Here's the drawing with two shaded views (mm, measured from the low corner). I have some questions. A direction names the side the tool comes from. Coordinates: 2 decimals unless noted, no trailing zeros. Loops run counter-clockwise (first coordinate to the right, second up) from the corner with the lowest first, then second, coordinate; pieces in that order, holes last. Notation, with made-up numbers: M 68.25,22.5 L 80.25,22.5 A18 cw 80.25,43.5 Z; hole C 10.25,-10 d8. An arc over 180 degrees is marked long. Return JSON: item names as keys, results as strings. Group by question number.
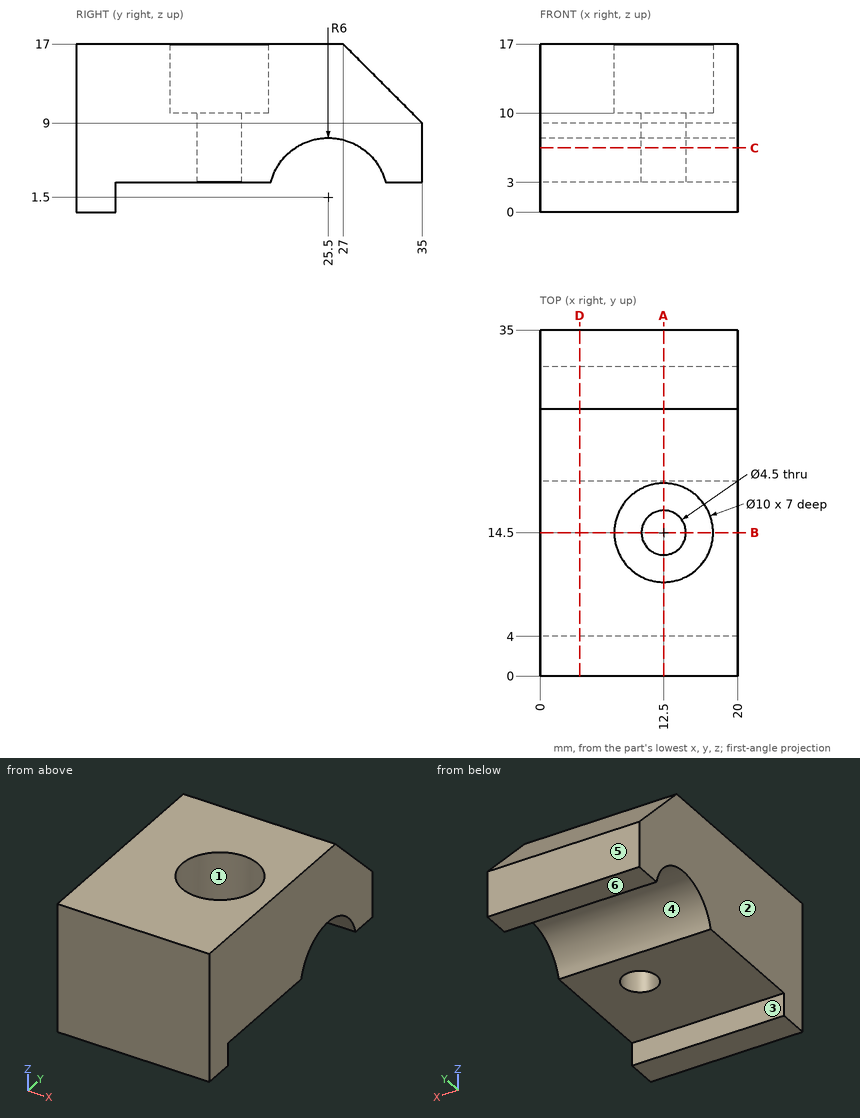
(1) Will these pins go through, and if not, where does the flat tip stop? P1, Ø3, axis at x = 15, y = 16.5, coming from the +Z side; P2, Ø4, axis at x = 9.5, y = 9, coming from the -Z side; P3, Ø3.5, axis at x = 7.5, z = 1, coming from the +Y side.
(2) If I drill on L1, parallel to Y at x = 11.25, z = 4.5; L2, parallel to Y at x = 15.5, z = 1; L3, parallel to Y at x = 18.75, z = 6.75, over which ranges is the centre line in solid material (lowest first)? Write a range as [from, to].
(3) Imagine slicing it at C-C, the plane z = 6.5. Write out the boundary of the cut face in (x, y).
(4) Imagine slicing it at D-D, the plane x = 4. Write out the boundary of the cut face in (y, z).
(5) Imagine slicing it at A-A, the plane x = 12.5. Write out the boundary of the cut face in (y, z), then the cut area to 3 significant figures.
(6) Imagine slicing it at B-B, the plane y = 14.5. Write out the boundary of the cut face in (x, z), then the cut area to 4 significant figures.
(7) We'd pull the mould along Y, two halves only. Please class the marked faces 4, 5 and 6: +Y half, -Y half, draft (parallel to the pull), parting line (faces both ways), or undercut.
(8) For the marked faces 1, 2 and 3, which set-ups out of +Z, -Z, +X, -X, +Y, -Y let a thin tool reach every point of the face, with its end or its side?
Checks:
{
 "1": {"P1": "z = 10", "P2": "z = 3", "P3": "y = 4"},
 "2": {"L1": "[0, 12.63], [16.37, 20.3], [30.7, 35]", "L2": "[0, 4]", "L3": "[0, 22.6], [28.4, 35]"},
 "3": {"outline": "M 0,0 L 20,0 L 20,22.18 L 0,22.18 Z; M 0,28.82 L 20,28.82 L 20,35 L 0,35 Z; hole C 12.5,14.5 d4.5"},
 "4": {"outline": "M 0,0 L 4,0 L 4,3 L 19.69,3 A6 cw 31.31,3 L 35,3 L 35,9 L 27,17 L 0,17 Z"},
 "5": {"outline": "M 0,0 L 4,0 L 4,3 L 12.25,3 L 12.25,10 L 9.5,10 L 9.5,17 L 0,17 Z; M 16.75,3 L 19.69,3 A6 cw 31.31,3 L 35,3 L 35,9 L 27,17 L 19.5,17 L 19.5,10 L 16.75,10 Z", "area": "330 mm²"},
 "6": {"outline": "M 0,3 L 10.25,3 L 10.25,10 L 7.5,10 L 7.5,17 L 0,17 Z; M 14.75,3 L 20,3 L 20,17 L 17.5,17 L 17.5,10 L 14.75,10 Z", "area": "178.5 mm²"},
 "7": {"face 4": "undercut", "face 5": "+Y half", "face 6": "draft"},
 "8": {"face 1": "+Z", "face 2": "+Z, -Z, -X, +Y, -Y", "face 3": "-Z, +X, -X, +Y"}
}
